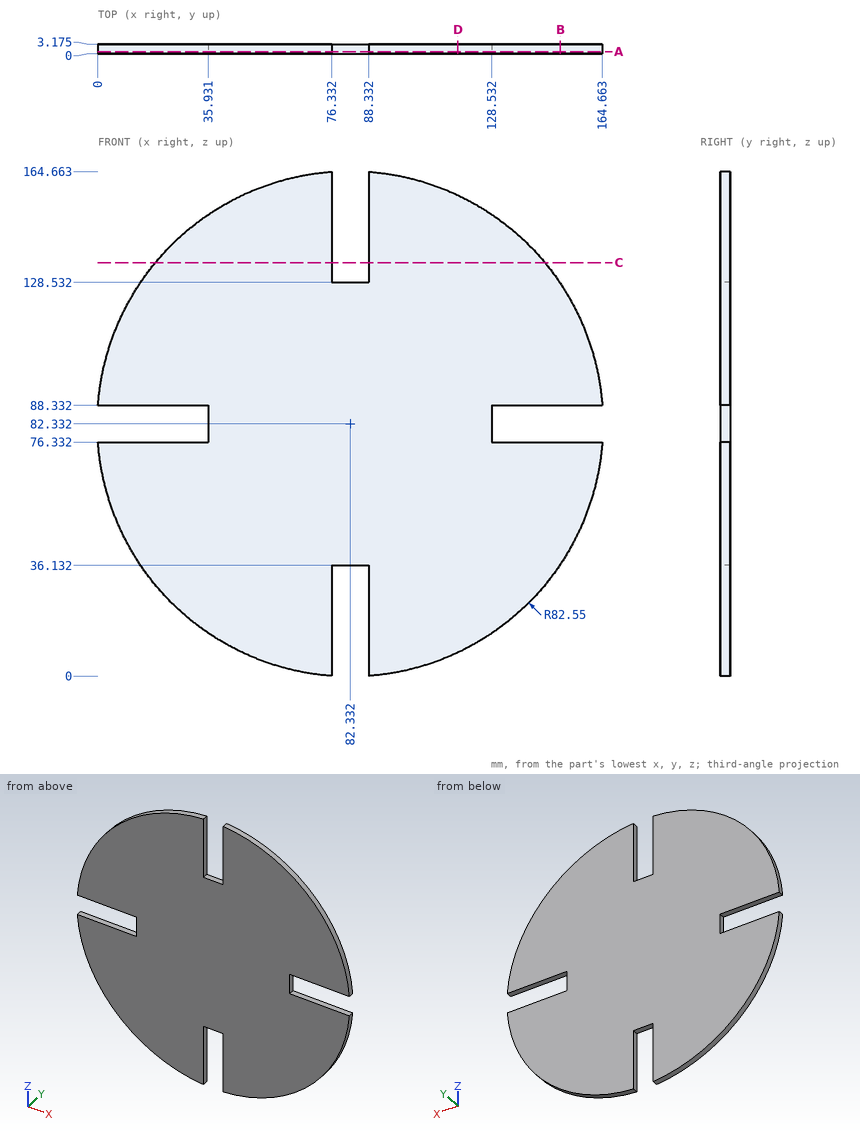
Here's the drawing with two shaded views (mm, measured from the low corner). I have some questions. Coordinates: 2 decimals unless noted, no trailing zeros. Write each loop counter-clockwise with the first axis right and the second up, starting at its lowest first coordinate (ties: lowest second). Pieces come first, ordered by that corner, then holes.
Item 1: I want a section at A-A on y = 0.65. Write out the boundary of the cut face in (x, z), and give its area (3 significant figures).
Item 2: I want a section at C-C on z = 135. Write out the boundary of the cut face in (x, y) (1 decimal).
Item 3: I want a section at D-D on x = 117.5. Write out the boundary of the cut face in (y, z) (1 decimal).
Item 4: I want a section at B-B on x = 151. Write out the boundary of the cut face in (y, z) (1 decimal).
Item 5: Will these pins go through, and if not, where does the flat tip stop? pin 1 (1.6 mm diameter, centred on y = 1, z = 17, fed in from -X); pin 2 (1.6 mm diameter, centred on y = 1.5, z = 12.5, fed in from +X); pin 3 (1 mm diameter, centred on x = 109.5, y = 2.5, fed in from +Z) (1 decimal).
Item 6: If I drill on line 1 (X direction, y = 0.85, z = 81); line 2 (X direction, y = 2.7, z = 149.5) (1 decimal); line 3 (X direction, y = 1.6, z = 34.5), over which ranges is the centre line in solid material (lowest first)?
Findings below:
1. outline: (0, 76.33) arc R82.55 ccw to (76.33, 0) - (76.33, 36.13) - (88.33, 36.13) - (88.33, 0) arc R82.55 ccw to (164.66, 76.33) - (128.53, 76.33) - (128.53, 88.33) - (164.66, 88.33) arc R82.55 ccw to (88.33, 164.66) - (88.33, 128.53) - (76.33, 128.53) - (76.33, 164.66) arc R82.55 ccw to (0, 88.33) - (35.93, 88.33) - (35.93, 76.33) - close
1. area: 19,700 mm2
2. outline: (18.8, 0) - (76.3, 0) - (76.3, 3.2) - (18.8, 3.2) - close; (88.3, 0) - (145.9, 0) - (145.9, 3.2) - (88.3, 3.2) - close
3. outline: (0, 7.6) - (3.2, 7.6) - (3.2, 157) - (0, 157) - close
4. outline: (0, 36.5) - (3.2, 36.5) - (3.2, 76.3) - (0, 76.3) - close; (0, 88.3) - (3.2, 88.3) - (3.2, 128.1) - (0, 128.1) - close
5. pin 1: stops at x = 30.85
5. pin 2: stops at x = 127.6
5. pin 3: stops at z = 160.5
6. line 1: x = 35.93 to 128.53
6. line 2: x = 34.3 to 76.3, 88.3 to 130.3
6. line 3: x = 15.05 to 76.33, 88.33 to 149.61
